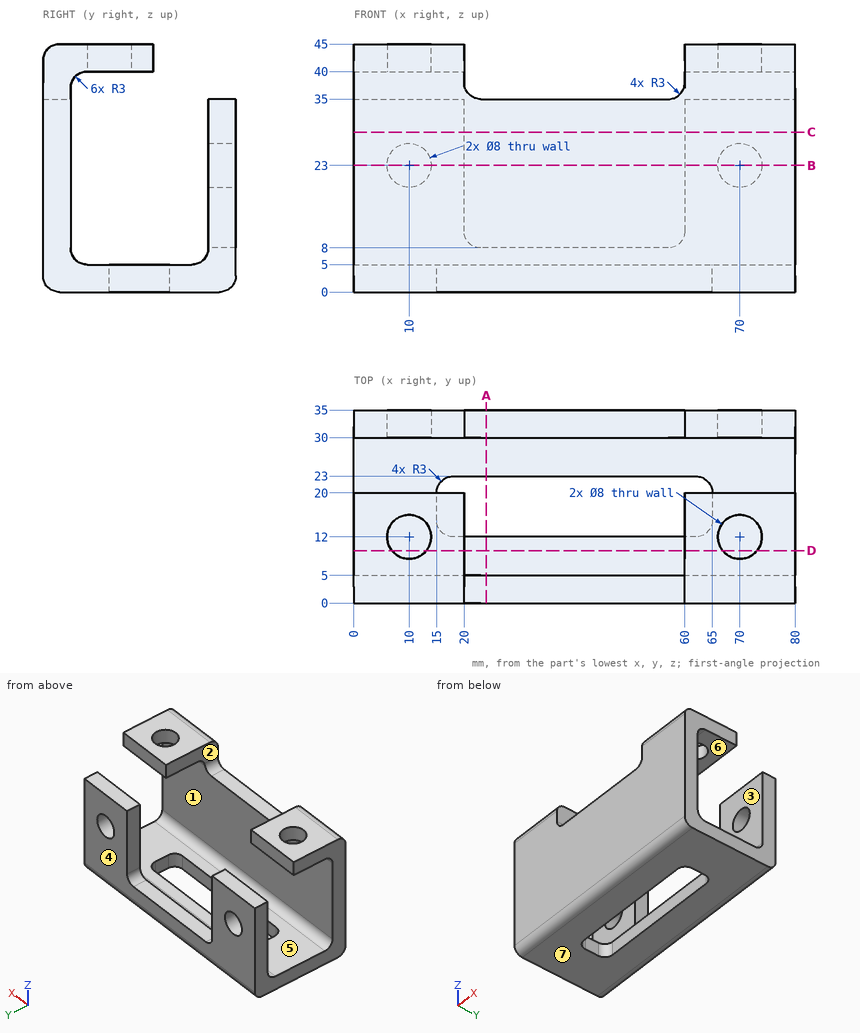
Input: dimensioned drawing with shaded views. Units: mm. Origin: part minimum x, y, z. A direction names the side the tool comes from. Give positions to 0.01 mm unless a question says otherwise; leave off trailing zeros. Loops run counter-clockwise (first coordinate to the right, second up) from the corner with the lowest first, then second, coordinate; pieces in that order, holes last. Notation, with made-up numbers: (31.25, -33) -> (63.25, -33) arc R14 cw to (63.25, -28) -> close; hole circle Ø4 at (22.25, 55). An arc over 180 degrees is marked (long way). Use a Markdown table: item, result.
Q1. Section query D-D, the plane y = 9.5. Return the cut outline in (x, z), plus the area to 3 significant figures.
Entries:
| item | result |
|---|---|
| outline | (0, 0) -> (80, 0) -> (80, 5) -> (0, 5) -> close; (0, 40) -> (6.88, 40) -> (6.88, 45) -> (0, 45) -> close; (13.12, 40) -> (20, 40) -> (20, 45) -> (13.12, 45) -> close; (60, 40) -> (66.88, 40) -> (66.88, 45) -> (60, 45) -> close; (73.12, 40) -> (80, 40) -> (80, 45) -> (73.12, 45) -> close |
| area | 538 mm² |
Q2. Ray query, probe 1 along X at (y, z) = (12, 43); probe 2 along Z at (x, y) = (10, 32); probe 3 along Z at (x, y) = (19, 9). Return the intervals inside material, ascending. Write a range as from..to.
Entries:
| item | result |
|---|---|
| probe 1 | x = 0..6, 14..20, 60..66, 74..80 |
| probe 2 | z = 0..19, 27..35 |
| probe 3 | z = 0..5, 40..45 |
Q3. Pull-direction query (Z, two-part tool) for the marked faces 4, 5, 6 and 7; classes: pulls with the +Z half, pulls with the -Z half, needs draft (parallel to the pull), parting line crosses it, or undercut.
Entries:
| item | result |
|---|---|
| face 4 | needs draft |
| face 5 | undercut |
| face 6 | undercut |
| face 7 | pulls with the -Z half |
Q4. Section query C-C, the plane z = 29. Return the cut outline in (x, y).
Entries:
| item | result |
|---|---|
| outline | (0, 0) -> (80, 0) -> (80, 5) -> (0, 5) -> close; (0, 30) -> (20, 30) -> (20, 35) -> (0, 35) -> close; (60, 30) -> (80, 30) -> (80, 35) -> (60, 35) -> close |
Q5. Access query for the marked faces 1, 2 and 3. Directions: +Z, -Z, +X, -X, +Y, -Y. A direction counts if a zero-diameter tool reaches every point of the face in a straight line with its end or side. Return the directions, or none.
Entries:
| item | result |
|---|---|
| face 1 | +X, -X |
| face 2 | +Z, +Y, -Y |
| face 3 | +Z, +X, -X |
Q6. First-contact query: P1, Ø2.5, axis at x = 44.5, y = 33.5, coming from the +Z side; P2, Ø3, axis at x = 45.5, y = 10, coming from the +Z side; P3, Ø12, axis at x = 63.5, y = 30, coming from the +Z side. Flat tips, straight axial feed; report the tip coordinate or a pass-through.
Entries:
| item | result |
|---|---|
| P1 | stops at z = 8 |
| P2 | stops at z = 5 |
| P3 | stops at z = 35 |
Q7. Section query B-B, the plane z = 23. Return the cut outline in (x, y).
Entries:
| item | result |
|---|---|
| outline | (0, 0) -> (80, 0) -> (80, 5) -> (0, 5) -> close; (0, 30) -> (6, 30) -> (6, 35) -> (0, 35) -> close; (14, 30) -> (20, 30) -> (20, 35) -> (14, 35) -> close; (60, 30) -> (66, 30) -> (66, 35) -> (60, 35) -> close; (74, 30) -> (80, 30) -> (80, 35) -> (74, 35) -> close |
Q8. Section query A-A, the plane x = 24. Return the cut outline in (y, z), plus the area to 3 significant figures.
Entries:
| item | result |
|---|---|
| outline | (0, 3) arc R3 ccw to (3, 0) -> (12, 0) -> (12, 5) -> (8, 5) arc R3 cw to (5, 8) -> (5, 35) -> (0, 35) -> close; (23, 0) -> (32, 0) arc R3 ccw to (35, 3) -> (35, 8) -> (30, 8) arc R3 cw to (27, 5) -> (23, 5) -> close |
| area | 285 mm² |
